Check sheet for the modelled part. Datum: model origin and axes. Units: mm. A direction names the side the tool comes from. Round coordinates to 2 decimals unless told otherwise and drop trailing zeros. Write each loop counter-clockwise with the first axis right and the second up, starting at its lowest first coordinate (ties: lowest second). Pieces come first, ordered by that corner, then holes.
Item 1: Section check C-C, the plane z = -985. Record the cut outline in (x, y), plus the area to 3 significant figures.
Item 2: Section check A-A, the plane y = 113. Record the cut outline in (x, z), plus the area to 3 significant figures.
Item 3: Section check B-B, the plane x = 347.5. Record the cut outline in (y, z).
Item 4: Material ranges on line 1 along X through (y, z) = (116.25, -989); line 2 along Z through (x, y) = (397, 115.25); line 3 along Y through (x, z) = (368, -968), recorded low to high.
Item 5: Depth check by flat-ended pin: pin 1 (2 mm diameter, centred on y = 115, z = -1057, fed in from +X); pin 2 (8 mm diameter, centred on x = 411.95, z = -952.22, fed in from -Y); pin 3 (4 mm diameter, centred on x = 241.95, z = -1052.22, fed in from +Y); pin 4 (2 mm diameter, centred on y = 115, z = -947, fed in from -X). Enter the tip coordinate at first touch or a pass-through.
Item 6: Set-up check for faces 5 (the cylindrical face through (247.31, 115.71, -1046.97)), 6 (the cylindrical face through (355.45, 117.71, -1022.12)): record each of +Z, -Z, +X, -X, +Y, -Y from which the full face is reachable in a straight line by a thin tool's end or side.
Item 7: Release check for a two-part mould opening along X. For faces 1 (the cylindrical face through (301.45, 117.71, -1022.12)), 2 (the flat face through (326, 117, -942.218)), 3 (the cylindrical face through (240.61, 117.71, -954.33)), 4 (the flat face through (231.951, 117, -1003)) record: pulls with the +X half, pulls with the -X half, needs draft (parallel to the pull), parting line crosses it, or undercut.
from build123d import *

# Parameters (mm, degrees)
SKETCH1_R                      = 5.5
BOSS_EXTRUDE1_DEPTH            = 5
BOSS_EXTRUDE2_DEPTH            = 2
SKETCH4_R                      = 1.4
BOSS_EXTRUDE3_DEPTH            = 7
SKETCH12_W                     = 20
SKETCH12_H                     = 2
CUT_EXTRUDE1_DEPTH             = 10
F_4_2_4_2_DIAMETER_HOLE1_D     = 4.2
F_4_2_4_2_DIAMETER_HOLE1_DEPTH = 20
F_4_2_4_2_DIAMETER_HOLE1_TIP   = 1.2618073
F_5_0_5_DIAMETER_HOLE1_D       = 5
F_5_0_5_DIAMETER_HOLE1_DEPTH   = 5
F_5_0_5_DIAMETER_HOLE1_TIP     = 1.502151548
SKETCH1_3_R                    = 5.5
CUT_EXTRUDE2_DEPTH             = 3


with BuildPart() as part:
    # Sketch1 → Boss-Extrude1 (new body)
    with BuildSketch(Plane(origin=(0, 111.722415865, 0), x_dir=(1, 0, 0), z_dir=(0, 1, 0))):
        with BuildLine():
            Line((241.95107426, 942.218289838), (411.95107426, 942.218289838))
            ThreePointArc((411.95107426, 942.218289838), (419.022142072, 945.147222026), (421.95107426, 952.218289838))
            Line((421.95107426, 952.218289838), (421.95107426, 1052.218289838))
            ThreePointArc((421.95107426, 1052.218289838), (419.022142072, 1059.28935765), (411.95107426, 1062.218289838))
            Line((411.95107426, 1062.218289838), (241.95107426, 1062.218289838))
            ThreePointArc((241.95107426, 1062.218289838), (234.880006448, 1059.28935765), (231.95107426, 1052.218289838))
            Line((231.95107426, 1052.218289838), (231.95107426, 952.218289838))
            ThreePointArc((231.95107426, 952.218289838), (234.880006448, 945.147222026), (241.95107426, 942.218289838))
        make_face()
        with Locations((241.95107426, 952.218289838)):
            Circle(SKETCH1_R, mode=Mode.SUBTRACT)
        with Locations((411.95107426, 952.218289838)):
            Circle(SKETCH1_R, mode=Mode.SUBTRACT)
        with Locations((411.95107426, 1052.218289838)):
            Circle(SKETCH1_R, mode=Mode.SUBTRACT)
        with Locations((241.95107426, 1052.218289838)):
            Circle(SKETCH1_R, mode=Mode.SUBTRACT)
        with BuildLine():
            Line((249.45107426, 952.218289838), (249.45107426, 944.718289838))
            Line((249.45107426, 944.718289838), (404.45107426, 944.718289838))
            Line((404.45107426, 944.718289838), (404.45107426, 952.218289838))
            ThreePointArc((404.45107426, 952.218289838), (406.647773401, 957.521590697), (411.95107426, 959.718289838))
            Line((411.95107426, 959.718289838), (419.45107426, 959.718289838))
            Line((419.45107426, 959.718289838), (419.45107426, 1044.718289838))
            Line((419.45107426, 1044.718289838), (411.95107426, 1044.718289838))
            ThreePointArc((411.95107426, 1044.718289838), (406.647773401, 1046.914988979), (404.45107426, 1052.218289838))
            Line((404.45107426, 1052.218289838), (404.45107426, 1059.718289838))
            Line((404.45107426, 1059.718289838), (249.45107426, 1059.718289838))
            Line((249.45107426, 1059.718289838), (249.45107426, 1052.218289838))
            ThreePointArc((249.45107426, 1052.218289838), (247.254375119, 1046.914988979), (241.95107426, 1044.718289838))
            Line((241.95107426, 1044.718289838), (234.45107426, 1044.718289838))
            Line((234.45107426, 1044.718289838), (234.45107426, 959.718289838))
            Line((234.45107426, 959.718289838), (241.95107426, 959.718289838))
            ThreePointArc((241.95107426, 959.718289838), (247.254375119, 957.521590697), (249.45107426, 952.218289838))
        make_face(mode=Mode.SUBTRACT)
    extrude(amount=BOSS_EXTRUDE1_DEPTH)

    # Sketch2 → Boss-Extrude2 (add)
    with BuildSketch(Plane(origin=(0, 116.722415865, 0), x_dir=(1, 0, 0), z_dir=(0, 1, 0))):
        with BuildLine():
            Line((231.95107426, 1052.218289838), (231.95107426, 952.218289838))
            ThreePointArc((231.95107426, 952.218289838), (234.880006448, 945.147222026), (241.95107426, 942.218289838))
            Line((241.95107426, 942.218289838), (411.95107426, 942.218289838))
            ThreePointArc((411.95107426, 942.218289838), (419.022142072, 945.147222026), (421.95107426, 952.218289838))
            Line((421.95107426, 952.218289838), (421.95107426, 1052.218289838))
            ThreePointArc((421.95107426, 1052.218289838), (419.022142072, 1059.28935765), (411.95107426, 1062.218289838))
            Line((411.95107426, 1062.218289838), (241.95107426, 1062.218289838))
            ThreePointArc((241.95107426, 1062.218289838), (234.880006448, 1059.28935765), (231.95107426, 1052.218289838))
        make_face()
    extrude(amount=BOSS_EXTRUDE2_DEPTH)

    # Sketch4 → Boss-Extrude3 (add)
    with BuildSketch(Plane(origin=(0, 118.722415865, 0), x_dir=(1, 0, 0), z_dir=(0, 1, 0))):
        with BuildLine():
            Line((375.86522753, 1030.272411662), (375.86522753, 1031.672411662))
            Line((375.86522753, 1031.672411662), (377.26522753, 1031.672411662))
            ThreePointArc((377.26522753, 1031.672411662), (374.875278036, 1032.662361156), (375.86522753, 1030.272411662))
        make_face()
        with BuildLine():
            Line((377.26522753, 1031.672411662), (375.86522753, 1031.672411662))
            Line((375.86522753, 1031.672411662), (375.86522753, 1030.272411662))
            ThreePointArc((375.86522753, 1030.272411662), (376.855177023, 1030.682462168), (377.26522753, 1031.672411662))
        make_face()
        with BuildLine():
            ThreePointArc((377.26522753, 1007.672411662), (376.855177023, 1008.662361156), (375.86522753, 1009.072411662))
            Line((375.86522753, 1009.072411662), (375.86522753, 1007.672411662))
            Line((375.86522753, 1007.672411662), (377.26522753, 1007.672411662))
        make_face()
        with BuildLine():
            Line((375.86522753, 1007.672411662), (375.86522753, 1009.072411662))
            ThreePointArc((375.86522753, 1009.072411662), (374.875278036, 1006.682462168), (377.26522753, 1007.672411662))
            Line((377.26522753, 1007.672411662), (375.86522753, 1007.672411662))
        make_face()
        with Locations((399.86522753, 1031.672411662)):
            Circle(SKETCH4_R)
        with Locations((399.86522753, 1007.672411662)):
            Circle(SKETCH4_R)
    extrude(amount=-BOSS_EXTRUDE3_DEPTH)

    # Sketch12 → Cut-Extrude1 (cut)
    with BuildSketch(Plane(origin=(0, 118.722415865, 0), x_dir=(1, 0, 0), z_dir=(0, 1, 0))):
        with Locations((328.108762335, 982.045276567)):
            Rectangle(SKETCH12_W, SKETCH12_H)
    extrude(amount=-CUT_EXTRUDE1_DEPTH, mode=Mode.SUBTRACT)

    # Ø4.2 (4.2) Diameter Hole1
    with Locations(Plane(origin=(0, 118.722415865, 0), x_dir=(1, 0, 0), z_dir=(0, 1, 0))):
        with Locations((300.990952506, 1024.17077451), (354.990952506, 1024.17077451), (354.990952506, 980.17077451), (300.990952506, 980.17077451)):
            Hole(F_4_2_4_2_DIAMETER_HOLE1_D / 2, depth=F_4_2_4_2_DIAMETER_HOLE1_DEPTH)
            with Locations((0, 0, -(F_4_2_4_2_DIAMETER_HOLE1_DEPTH + F_4_2_4_2_DIAMETER_HOLE1_TIP / 2))):  # 118° drill point
                Cone(0, F_4_2_4_2_DIAMETER_HOLE1_D / 2, F_4_2_4_2_DIAMETER_HOLE1_TIP, mode=Mode.SUBTRACT)

    # Ø5.0 (5) Diameter Hole1
    with Locations(Plane(origin=(0, 118.722415865, 0), x_dir=(1, 0, 0), z_dir=(0, 1, 0))):
        with Locations((241.95107426, 1052.218289838), (411.95107426, 1052.218289838), (411.95107426, 952.218289838), (241.95107426, 952.218289838)):
            Hole(F_5_0_5_DIAMETER_HOLE1_D / 2, depth=F_5_0_5_DIAMETER_HOLE1_DEPTH)
            with Locations((0, 0, -(F_5_0_5_DIAMETER_HOLE1_DEPTH + F_5_0_5_DIAMETER_HOLE1_TIP / 2))):  # 118° drill point
                Cone(0, F_5_0_5_DIAMETER_HOLE1_D / 2, F_5_0_5_DIAMETER_HOLE1_TIP, mode=Mode.SUBTRACT)

    # Sketch1<3> → Cut-Extrude2 (cut)
    with BuildSketch(Plane(origin=(0, 111.722415865, 0), x_dir=(1, 0, 0), z_dir=(0, 1, 0))):
        with BuildLine():
            Line((241.95107426, 942.218289838), (411.95107426, 942.218289838))
            ThreePointArc((411.95107426, 942.218289838), (419.022142072, 945.147222026), (421.95107426, 952.218289838))
            Line((421.95107426, 952.218289838), (421.95107426, 1052.218289838))
            ThreePointArc((421.95107426, 1052.218289838), (419.022142072, 1059.28935765), (411.95107426, 1062.218289838))
            Line((411.95107426, 1062.218289838), (241.95107426, 1062.218289838))
            ThreePointArc((241.95107426, 1062.218289838), (234.880006448, 1059.28935765), (231.95107426, 1052.218289838))
            Line((231.95107426, 1052.218289838), (231.95107426, 952.218289838))
            ThreePointArc((231.95107426, 952.218289838), (234.880006448, 945.147222026), (241.95107426, 942.218289838))
        make_face()
        with Locations((241.95107426, 952.218289838)):
            Circle(SKETCH1_3_R, mode=Mode.SUBTRACT)
        with Locations((411.95107426, 952.218289838)):
            Circle(SKETCH1_3_R, mode=Mode.SUBTRACT)
        with Locations((411.95107426, 1052.218289838)):
            Circle(SKETCH1_3_R, mode=Mode.SUBTRACT)
        with Locations((241.95107426, 1052.218289838)):
            Circle(SKETCH1_3_R, mode=Mode.SUBTRACT)
        with BuildLine():
            Line((249.45107426, 952.218289838), (249.45107426, 944.718289838))
            Line((249.45107426, 944.718289838), (404.45107426, 944.718289838))
            Line((404.45107426, 944.718289838), (404.45107426, 952.218289838))
            ThreePointArc((404.45107426, 952.218289838), (406.647773401, 957.521590697), (411.95107426, 959.718289838))
            Line((411.95107426, 959.718289838), (419.45107426, 959.718289838))
            Line((419.45107426, 959.718289838), (419.45107426, 1044.718289838))
            Line((419.45107426, 1044.718289838), (411.95107426, 1044.718289838))
            ThreePointArc((411.95107426, 1044.718289838), (406.647773401, 1046.914988979), (404.45107426, 1052.218289838))
            Line((404.45107426, 1052.218289838), (404.45107426, 1059.718289838))
            Line((404.45107426, 1059.718289838), (249.45107426, 1059.718289838))
            Line((249.45107426, 1059.718289838), (249.45107426, 1052.218289838))
            ThreePointArc((249.45107426, 1052.218289838), (247.254375119, 1046.914988979), (241.95107426, 1044.718289838))
            Line((241.95107426, 1044.718289838), (234.45107426, 1044.718289838))
            Line((234.45107426, 1044.718289838), (234.45107426, 959.718289838))
            Line((234.45107426, 959.718289838), (241.95107426, 959.718289838))
            ThreePointArc((241.95107426, 959.718289838), (247.254375119, 957.521590697), (249.45107426, 952.218289838))
        make_face(mode=Mode.SUBTRACT)
    extrude(amount=CUT_EXTRUDE2_DEPTH, mode=Mode.SUBTRACT)


solid = part.part
Values found:
1. outline: (231.95, 114.72) - (234.45, 114.72) - (234.45, 116.72) - (419.45, 116.72) - (419.45, 114.72) - (421.95, 114.72) - (421.95, 118.72) - (231.95, 118.72) - close
1. area: 390 mm2
2. outline: circle Ø2.8 at (375.87, -1031.67); circle Ø2.8 at (375.87, -1007.67); circle Ø2.8 at (399.87, -1031.67); circle Ø2.8 at (399.87, -1007.67)
2. area: 24.6 mm2
3. outline: (114.72, -1062.22) - (118.72, -1062.22) - (118.72, -942.22) - (114.72, -942.22) - (114.72, -944.72) - (116.72, -944.72) - (116.72, -1059.72) - (114.72, -1059.72) - close
4. line 1: x = 231.95 to 234.45, 419.45 to 421.95
4. line 2: z = -1062.22 to -1059.72, -944.72 to -942.22
4. line 3: y = 116.72 to 118.72
5. pin 1: stops at x = 421.21
5. pin 2: stops at y = 116.72
5. pin 3: passes through
5. pin 4: stops at x = 232.88
6. face 5: -Y
6. face 6: +Y, -Y
7. face 1: undercut
7. face 2: needs draft
7. face 3: undercut
7. face 4: pulls with the -X half
